from build123d import *

# Parameters (mm, degrees)
F1_DEPTH       = 2.75
F2_DEPTH       = 17.75
F4_D           = 3.3
F4_CSINK_D     = 6.72
F4_CSINK_ANGLE = 90
F6_DEPTH       = 15
F7_R           = 2


with BuildPart() as f1:
    # F0 (on Front) → F1 (new body)
    with BuildSketch(Plane.XZ):
        Polygon((13.5, 52.5), (0, 52.5), (-13.5, 52.5), (-24, 23.5), (-13.5, -5.5), (0, -5.5), (13.5, -5.5), (24, 23.5), align=None)
        Polygon((13.5, 0), (0, 0), (-13.5, 0), (-13.5, 41), (-7.5, 47), (0, 47), (7.5, 47), (13.5, 41), align=None, mode=Mode.SUBTRACT)
        Polygon((-13.5, 0), (0, 0), (13.5, 0), (13.5, 41), (7.5, 47), (0, 47), (-7.5, 47), (-13.5, 41), align=None)
    extrude(amount=F1_DEPTH)

    # F0 (on Front) → F2 (join)
    with BuildSketch(Plane.XZ):
        Polygon((-13.5, 0), (0, 0), (13.5, 0), (13.5, 41), (7.5, 47), (0, 47), (-7.5, 47), (-13.5, 41), align=None)
    extrude(amount=-F2_DEPTH)

    # F4 (through all)
    with Locations(Plane.XZ.offset(2.75)):
        with Locations((-19.9, 23.5), (19.9, 23.5)):
            CounterSinkHole(F4_D / 2, F4_CSINK_D / 2, counter_sink_angle=F4_CSINK_ANGLE)

    # F5 (on face) → F6 (cut)
    with BuildSketch(Plane.XZ.offset(2.75)):
        Polygon((7, 45.5), (0, 45.5), (-7, 45.5), (-12, 40.5), (-12, 29.2), (0, 29.2), (12, 29.2), (12, 40.5), align=None)
    extrude(amount=-F6_DEPTH, mode=Mode.SUBTRACT)

    # F7
    f7_edges = [f1.edges().sort_by_distance(p)[0] for p in [
        (13.5, -1.375, 52.5),
        (-13.5, -1.375, 52.5),
        (-7.5, 8.875, 47),
        (-13.5, 8.875, 41),
        (7.5, 8.875, 47),
        (13.5, 8.875, 41),
        (-24, -1.375, 23.5),
        (-13.5, -1.375, -5.5),
        (13.5, -1.375, -5.5),
        (24, -1.375, 23.5),
        (13.5, 8.875, 0),
        (-13.5, 8.875, 0),
        (-12, 4.75, 29.2),
        (12, 4.75, 29.2),
        (12, 4.75, 40.5),
        (7, 4.75, 45.5),
        (-12, 4.75, 40.5),
        (-7, 4.75, 45.5),
    ]]
    fillet(f7_edges, radius=F7_R)


solid = f1.part
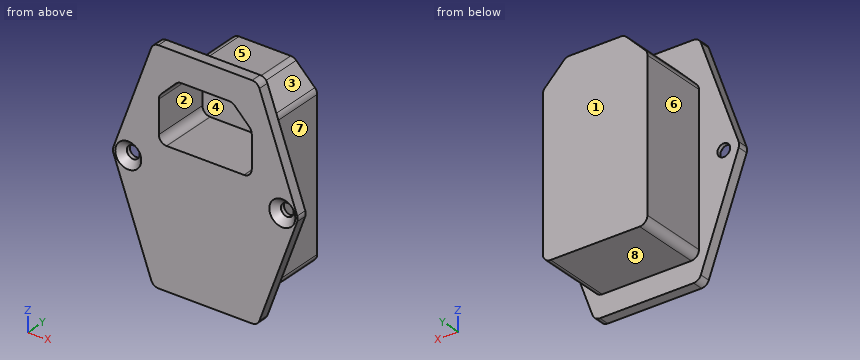
Source: CAD feature listing. Evaluate the final solid. Frame: model axes, mm. Face numbers are marked on the shaded views. A direction names the side the tool comes from. Coordinates: 2 decimals unless noted, no trailing zeros. Order: outer loops, then holes, each group sorted by start corner. A loop starts at its lowest first (then second) coordinate and runs counter-clockwise, first axis right, second up.
Item 1: Material intervals for line 1 (Z direction, x = 2.5, y = 1.5); line 2 (X direction, y = 3.75, z = 34.5); line 3 (Y direction, x = 2.5, z = 44), sorted ascending.
Output values:
line 1: z = 0 to 29.2, 45.5 to 47
line 2: x = -13.5 to -12, 12 to 13.5
line 3: y = 12.25 to 17.75
Item 2: Cut plane D-D (y = 13.25). Return loops of the section in (x, z).
Output values:
outline: (-13.5, 2) arc R2 ccw to (-11.5, 0) - (11.5, 0) arc R2 ccw to (13.5, 2) - (13.5, 40.17) arc R2 ccw to (12.91, 41.59) - (8.09, 46.41) arc R2 ccw to (6.67, 47) - (-6.67, 47) arc R2 ccw to (-8.09, 46.41) - (-12.91, 41.59) arc R2 ccw to (-13.5, 40.17) - close
Item 3: Cut plane B-B (y = 8.5). Return loops of the section in (x, z), plus the area to 3 significant figures.
Output values:
outline: (-13.5, 2) arc R2 ccw to (-11.5, 0) - (11.5, 0) arc R2 ccw to (13.5, 2) - (13.5, 40.17) arc R2 ccw to (12.91, 41.59) - (8.09, 46.41) arc R2 ccw to (6.67, 47) - (-6.67, 47) arc R2 ccw to (-8.09, 46.41) - (-12.91, 41.59) arc R2 ccw to (-13.5, 40.17) - close; hole (-12, 31.2) arc R2 ccw to (-10, 29.2) - (10, 29.2) arc R2 ccw to (12, 31.2) - (12, 39.67) arc R2 ccw to (11.41, 41.09) - (7.59, 44.91) arc R2 ccw to (6.17, 45.5) - (-6.17, 45.5) arc R2 ccw to (-7.59, 44.91) - (-11.41, 41.09) arc R2 ccw to (-12, 39.67) - close
area: 867 mm2
Item 4: Cut plane C-C (x = 19.9). Return loops of the section in (y, z).
Output values:
outline: (-2.75, 12.18) - (0, 12.18) - (0, 21.85) - (-1.04, 21.85) - (-2.75, 20.14) - close; (-2.75, 26.86) - (-1.04, 25.15) - (0, 25.15) - (0, 34.82) - (-2.75, 34.82) - close
Item 5: Set-up query: the marked faces 4, 5, 6, 7 and 8. Return all of +Z, -Z, +X, -X, +Y, -Y with unobstructed straight access to the full face (end or side cutting, diameter ignored); none if empty.
Output values:
face 4: -Y
face 5: +Z, +X, -X, +Y
face 6: +Z, -Z, -X, +Y
face 7: +Z, -Z, +X, +Y
face 8: -Z, +X, -X, +Y
Item 6: Pull-direction query (Z, two-part tool) for the marked faces 1, 2 and 3; classes: pulls with the +Z half, pulls with the -Z half, needs draft (parallel to the pull), parting line crosses it, or undercut.
Output values:
face 1: needs draft
face 2: undercut
face 3: pulls with the +Z half
Item 7: First-contact query: P1, Ø2.5, axis at y = 8, z = 33.5, coming from the +X side; P2, Ø3.5, axis at x = 0, y = 5.5, coming from the -Z side; P3, Ø1, axis at y = 14, z = 4, coming from the -X side. Flat tips, straight axial feed; report the tip coordinate or a pass-through.
Output values:
P1: stops at x = 13.5
P2: stops at z = 0
P3: stops at x = -13.5
Item 8: Cut plane A-A (z = 23.5). Return loops of the section in (x, y), plus the area to 3 significant figures.
Output values:
outline: (-23.87, -2.75) - (-23.26, -2.75) - (-21.55, -1.04) - (-21.55, 0) - (-23.87, 0) - close; (-18.25, -1.04) - (-16.54, -2.75) - (16.54, -2.75) - (18.25, -1.04) - (18.25, 0) - (13.5, 0) - (13.5, 17.75) - (-13.5, 17.75) - (-13.5, 0) - (-18.25, 0) - close; (21.55, -1.04) - (23.26, -2.75) - (23.87, -2.75) - (23.87, 0) - (21.55, 0) - close
area: 587 mm2
